from build123d import *

# Parameters (mm, degrees)
SKETCH1_R              = 7.5
SKETCH1_R_2            = 1.25
BOSS_EXTRUDE1_DEPTH    = 3
FILLET1_R              = 3
SKETCH4_W              = 3
SKETCH4_H              = 175
BOSS_EXTRUDE3_DEPTH    = 27
SKETCH5_R              = 1.25
CUT_EXTRUDE2_DEPTH     = 212.917436753
FILLET4_R              = 2
SKETCH12_W             = 3
SKETCH12_H             = 90
BOSS_EXTRUDE5_DEPTH    = 12.5
CUT_EXTRUDE1_START     = -22
SKETCH2_R              = 2.4
CUT_EXTRUDE1_DEPTH     = 192.365882934
CUT_EXTRUDE8_DEPTH     = 214.365882934
FILLET5_R              = 2
SKETCH51_R             = 1.25
CUT_EXTRUDE9_DEPTH     = 214.365882934
CONVERT_SOLID9_START   = 110
CONVERT_SOLID9_DEPTH   = 90
CONVERT_SOLID9_2_DEPTH = 90


# Read off the part's stored shape, not the designer's step: Convert-Solid9
with BuildPart() as part:
    # Sketch1 → Boss-Extrude1 (new body)
    with BuildSketch(Plane(origin=(0, 0, 0), x_dir=(0, 0, -1), z_dir=(1, 0, 0))):
        with BuildLine():
            Line((-30, -16.155216865), (-30, 1))
            Line((-30, 1), (-35, 15))
            Line((-35, 15), (-35, 25))
            Line((-35, 25), (-62, 25))
            Line((-62, 25), (-62, 15))
            Line((-62, 15), (-69.665068474, -26.355129371))
            ThreePointArc((-69.665068474, -26.355129371), (-55.754353698, -49.154305352), (-31.582037919, -37.796067776))
            Line((-31.582037919, -37.796067776), (-9.457329759, -41.697250765))
            Line((-9.457329759, -41.697250765), (-6.856499335, -26.947208462))
            Line((-6.856499335, -26.947208462), (-30, -16.155216865))
        make_face()
        with Locations((-50, -30)):
            Circle(SKETCH1_R, mode=Mode.SUBTRACT)
        with Locations((-23.361205166, -34.168489335)):
            Circle(SKETCH1_R_2, mode=Mode.SUBTRACT)
        with Locations((-13.513127636, -35.904971111)):
            Circle(SKETCH1_R_2, mode=Mode.SUBTRACT)
    extrude(amount=BOSS_EXTRUDE1_DEPTH)

    # Fillet1
    fillet1_edges = [part.edges().sort_by_distance(p)[0] for p in [
        (1.5, 15, 35),
        (1.5, 1, 30),
        (1.5, -16.155216865, 30),
        (1.5, -26.947208462, 6.856499335),
        (1.5, -41.697250765, 9.457329759),
        (1.5, -37.796067776, 31.582037919),
        (1.5, 15, 62),
    ]]
    fillet(fillet1_edges, radius=FILLET1_R)

    # Sketch4 → Boss-Extrude3 (add)
    with BuildSketch(Plane(origin=(0, 0, 35), x_dir=(-1, 0, 0), z_dir=(0, 0, -1))):
        with Locations((-1.5, 112.5)):
            Rectangle(SKETCH4_W, SKETCH4_H)
    extrude(amount=-BOSS_EXTRUDE3_DEPTH)

    # Sketch5 → Cut-Extrude2 (cut, through all)
    with BuildSketch(Plane.ZY):
        with Locations((48.5, 185)):
            Circle(SKETCH5_R)
        with Locations((48.5, 115)):
            Circle(SKETCH5_R)
    extrude(amount=-CUT_EXTRUDE2_DEPTH, mode=Mode.SUBTRACT)

    # Fillet4
    fillet4_edges = [part.edges().sort_by_distance(p)[0] for p in [
        (1.5, 200, 35),
    ]]
    fillet(fillet4_edges, radius=FILLET4_R)

    # Sketch12 → Boss-Extrude5 (add)
    with BuildSketch(Plane(origin=(3, 0, 0), x_dir=(0, 0, -1), z_dir=(1, 0, 0))):
        with Locations((-63.5, 155)):
            Rectangle(SKETCH12_W, SKETCH12_H)
    extrude(amount=-BOSS_EXTRUDE5_DEPTH)

    # Mirror2: part across plane


with BuildPart() as part_1:
    add(part.part)
    add(part.part.mirror(Plane.ZY.offset(9.5)))

    # Sketch2 → Cut-Extrude1 (cut, through all)
    with BuildSketch(Plane(origin=(3, 0, 0), x_dir=(0, 0, -1), z_dir=(1, 0, 0)).offset(CUT_EXTRUDE1_START)):
        with Locations(Location((-62.688309019, -35.916655664, 0), (0, 0, 180))):
            Circle(SKETCH2_R)
    extrude(amount=-CUT_EXTRUDE1_DEPTH, mode=Mode.SUBTRACT)

    # Sketch50 → Cut-Extrude8 (cut, through all)
    with BuildSketch(Plane(origin=(3, 0, 0), x_dir=(0, 0, -1), z_dir=(1, 0, 0))):
        with BuildLine():
            Line((-62, 110), (-57, 110))
            ThreePointArc((-57, 110), (-56, 109), (-57, 108))
            Line((-57, 108), (-62, 108))
            Line((-62, 108), (-62, 110))
        make_face()
    extrude(amount=-CUT_EXTRUDE8_DEPTH, mode=Mode.SUBTRACT)

    # Fillet5
    fillet5_edges = [part_1.edges().sort_by_distance(p)[0] for p in [
        (1.5, 108, 62),
        (-20.5, 108, 62),
    ]]
    fillet(fillet5_edges, radius=FILLET5_R)

    # Sketch51 → Cut-Extrude9 (cut, through all)
    with BuildSketch(Plane.ZY.offset(22)):
        with Locations((50, -10)):
            Circle(SKETCH51_R)
    extrude(amount=-CUT_EXTRUDE9_DEPTH, mode=Mode.SUBTRACT)

    # Convert-Solid9 outline → Convert-Solid9 (cut)
    with BuildSketch(Plane(origin=(0, 0, 0), x_dir=(1, 0, 0), z_dir=(0, 1, 0)).offset(CONVERT_SOLID9_START)):
        with BuildLine():
            Line((-3, -65), (3, -65))
            Line((3, -65), (3, -59))
            ThreePointArc((3, -59), (1.242640687, -63.242640687), (-3, -65))
        make_face()
        with BuildLine():
            Line((-22, -65), (-16, -65))
            ThreePointArc((-16, -65), (-20.242640687, -63.242640687), (-22, -59))
            Line((-22, -59), (-22, -65))
        make_face()
    extrude(amount=CONVERT_SOLID9_DEPTH, mode=Mode.SUBTRACT)

    # Convert-Solid9 2 outline → Convert-Solid9 2 (add)
    with BuildSketch(Plane(origin=(0, 0, 0), x_dir=(1, 0, 0), z_dir=(0, 1, 0)).offset(CONVERT_SOLID9_START)):
        with BuildLine():
            Line((0, -62), (0, -59))
            ThreePointArc((0, -59), (-0.878679656, -61.121320344), (-3, -62))
            Line((-3, -62), (0, -62))
        make_face()
        with BuildLine():
            Line((-19, -62), (-16, -62))
            ThreePointArc((-16, -62), (-18.121320344, -61.121320344), (-19, -59))
            Line((-19, -59), (-19, -62))
        make_face()
    extrude(amount=CONVERT_SOLID9_2_DEPTH)


solid = part_1.part
Can you work these out from the model? Positions are in its coordinate system, mm. A direction names the side the tool comes from. Give positions to 0.01 mm unless a question says otherwise; leave off trailing zeros. Loops run counter-clockwise (first coordinate to the right, second up) from the corner with the lowest first, then second, coordinate; pieces in that order, holes last. Notation, with made-up numbers: (36.5, 45.5) - (89.5, 45.5) arc R16 ccw to (89.5, 56.5) - close; hole circle Ø2 at (44.5, 58.25). An arc over 180 degrees is marked (long way). Answer as a JSON object with one key per item and string values.
Q1. Imagine slicing it at B-B on z = 18. Write out the boundary of the cut face in (x, y).
Geometry says:
{"outline": "(-22, -40.19) - (-19, -40.19) - (-19, -21.75) - (-22, -21.75) - close; (0, -40.19) - (3, -40.19) - (3, -21.75) - (0, -21.75) - close"}
Q2. If we mould it in two halves opening along Z, with no side actions, what happens to faces 6 (the flat face through (-20.5, -5.5, 65.8)), 7 (the flat face through (0, 45, 45)), 8 (the cylindrical face through (-20.48, -37.54, 60.92))? For each: pulls with the +Z half, pulls with the -Z half, needs draft (parallel to the pull), parting line crosses it, or undercut.
Geometry says:
{"face 6": "pulls with the +Z half", "face 7": "needs draft", "face 8": "undercut"}
Q3. Imagine slicing it at A-A on y = 30.5. Write out the boundary of the cut face in (x, z), plus the area to 3 significant figures.
Geometry says:
{"outline": "(-22, 35) - (-19, 35) - (-19, 62) - (-22, 62) - close; (0, 35) - (3, 35) - (3, 62) - (0, 62) - close", "area": "162 mm²"}
Q4. If I drill on L1, parallel to X at y = -30, z = 20.5; L2, parallel to Y at x = -21, z = 48.5; L3, parallel to Z at x = -11.5, y = 123, over which ranges is the centre line in solid material (lowest first)?
Geometry says:
{"L1": "-22 to -19, 0 to 3", "L2": "-49.94 to -37.35, -22.65 to 113.75, 116.25 to 183.75, 186.25 to 200", "L3": "62 to 65"}
Q5. Which directions (+Z, -Z, +X, -X, +Y, -Y) give clear straight access to the entire face, cutting with the end or side of a thin tool? Please do faces 1 (the cylindrical face through (-20.196, 154.37, 63.289)), 2 (the cylindrical face through (1.289, 154.37, 63.196)), 3 (the flat face through (3, 49, 46)), 4 (the flat face through (-10, 110, 63)), 5 (the flat face through (-10, 154, 62)).
Geometry says:
{"face 1": "+Z, -X, +Y", "face 2": "+Z, +X, +Y", "face 3": "+Z, -Z, +X, +Y, -Y", "face 4": "+Z, +X, -X", "face 5": "-Z, +Y, -Y"}
Q6. Will these pins go through, and if not, where does the flat tip stop? P1, Ø1, axis at x = -4, y = 166, coming from the +Z side; P2, Ø3, axis at y = -10, z = 50, coming from the -X side; P3, Ø10, axis at x = -17.5, z = 56.5, coming from the -Y side (3 decimals); P4, Ø1.5, axis at x = -21, y = 72.5, coming from the -Z side.
Geometry says:
{"P1": "z = 65", "P2": "x = -22", "P3": "y = -49.925", "P4": "z = 35"}
